from build123d import *

# Parameters (mm, degrees)
SKETCH1_W                                           = 125
SKETCH1_H                                           = 20
BOSS_EXTRUDE1_DEPTH                                 = 32
SKETCH2_R                                           = 6.4897
CUT_EXTRUDE1_DEPTH                                  = 4
SKETCH3_R                                           = 6.5
CUT_EXTRUDE2_DEPTH                                  = 6.5
CUT_EXTRUDE4_REACH                                  = 132.572
SKETCH8_R                                           = 2.1
SKETCH9_R                                           = 2.825
CUT_EXTRUDE5_DEPTH                                  = 1.1
M3X0_5_TAPPED_HOLE1_AT_2_COUNT                      = 2
M3X0_5_TAPPED_HOLE1_AT_2_PITCH                      = 14
LPATTERN1_COUNT                                     = 5
LPATTERN1_PITCH                                     = 25
M2_TAPPED_HOLE1_REACH                               = 132.572
M2_TAPPED_HOLE1_BORE_R                              = 0.8
CBORE_FOR_M6_HEX_SOCKET_HEAD_CAP_SCREW1_D           = 6.2
CBORE_FOR_M6_HEX_SOCKET_HEAD_CAP_SCREW1_CBORE_D     = 10.5
CBORE_FOR_M6_HEX_SOCKET_HEAD_CAP_SCREW1_CBORE_DEPTH = 4


with BuildPart() as part:
    # Sketch1 → Boss-Extrude1 (new body)
    with BuildSketch(Plane(origin=(0, 0, 0), x_dir=(1, 0, 0), z_dir=(0, 1, 0))):
        with Locations((62.5, 10)):
            Rectangle(SKETCH1_W, SKETCH1_H)
    extrude(amount=BOSS_EXTRUDE1_DEPTH)

    # Sketch2 → Cut-Extrude1 (cut)
    with BuildSketch(Plane.XY):
        with Locations((12.5, 16)):
            Circle(SKETCH2_R)
    cut_extrude1 = extrude(amount=-CUT_EXTRUDE1_DEPTH, mode=Mode.SUBTRACT)

    # Sketch3 → Cut-Extrude2 (cut)
    with BuildSketch(Plane.XY.offset(-4)):
        with Locations((12.5, 16)):
            Circle(SKETCH3_R)
    cut_extrude2 = extrude(amount=-CUT_EXTRUDE2_DEPTH, mode=Mode.SUBTRACT)

    # Sketch6 → M12x0.5 Tapped Hole1 (revolve, cut)
    with BuildSketch(Plane(origin=(12.5, 16, -10.5), x_dir=(0, -1, 0), z_dir=(1, 0, 0))):
        Polygon((0, 0), (0, 7.454948559), (5.75, 4), (5.75, 0), align=None)
    m12x0_5_tapped_hole1 = revolve(axis=Axis((12.5, 16, -4.15), (0, 0, -1)), mode=Mode.SUBTRACT)

    # Sketch8 → Cut-Extrude4 (cut, up to next)
    with BuildSketch(Plane.XY, mode=Mode.PRIVATE) as cut_extrude4_sk1:
        with Locations((12.5, 16)):
            Circle(SKETCH8_R)
    cut_extrude4_tool1 = extrude(cut_extrude4_sk1.sketch, amount=-CUT_EXTRUDE4_REACH, mode=Mode.PRIVATE) & part.part
    cut_extrude4 = cut_extrude4_tool1.solids().sort_by_distance((12.5, 16, 0))[0]
    add(cut_extrude4, mode=Mode.SUBTRACT)

    # Sketch9 → Cut-Extrude5 (cut)
    with BuildSketch(Plane(origin=(0, 0, -20), x_dir=(-1, 0, 0), z_dir=(0, 0, -1))):
        with Locations((-12.5, 16)):
            Circle(SKETCH9_R)
    cut_extrude5 = extrude(amount=-CUT_EXTRUDE5_DEPTH, mode=Mode.SUBTRACT)

    # Sketch11 → M3x0.5 Tapped Hole1 (revolve, cut)
    with BuildSketch(Plane(origin=(19.5, 16, -20), x_dir=(0, 1, 0), z_dir=(1, 0, 0))):
        Polygon((0, 0), (0, 5.251075774), (1.25, 4.5), (1.25, 0), align=None)
    m3x0_5_tapped_hole1 = revolve(axis=Axis((19.5, 16, -26.35), (0, 0, 1)), mode=Mode.SUBTRACT)

    # M3x0.5 Tapped Hole1 at 2: M3x0.5 Tapped Hole1 ×2
    with Locations(*[(-i * M3X0_5_TAPPED_HOLE1_AT_2_PITCH, 0, 0) for i in range(1, M3X0_5_TAPPED_HOLE1_AT_2_COUNT)]):
        add(m3x0_5_tapped_hole1, mode=Mode.SUBTRACT)

    # LPattern1: Cut-Extrude1, Cut-Extrude2, M12x0.5 Tapped Hole1, Cut-Extrude4, Cut-Extrude5, M3x0.5 Tapped Hole1 ×5
    with Locations(*[(i * LPATTERN1_PITCH, 0, 0) for i in range(1, LPATTERN1_COUNT)]):
        add(cut_extrude1, mode=Mode.SUBTRACT)
        add(cut_extrude2, mode=Mode.SUBTRACT)
        add(m12x0_5_tapped_hole1, mode=Mode.SUBTRACT)
        add(cut_extrude4, mode=Mode.SUBTRACT)
        add(cut_extrude5, mode=Mode.SUBTRACT)
        add(m3x0_5_tapped_hole1, mode=Mode.SUBTRACT)

    # LPattern1 copy 1 sketch → LPattern1 copy 1 (revolve, cut)
    with BuildSketch(Plane(origin=(30.5, 16, -20), x_dir=(0, 1, 0), z_dir=(1, 0, 0))):
        Polygon((0, 0), (0, 5.251075774), (1.25, 4.5), (1.25, 0), align=None)
    revolve(axis=Axis((30.5, 16, -26.35), (0, 0, 1)), mode=Mode.SUBTRACT)

    # LPattern1 copy 2 sketch → LPattern1 copy 2 (revolve, cut)
    with BuildSketch(Plane(origin=(55.5, 16, -20), x_dir=(0, 1, 0), z_dir=(1, 0, 0))):
        Polygon((0, 0), (0, 5.251075774), (1.25, 4.5), (1.25, 0), align=None)
    revolve(axis=Axis((55.5, 16, -26.35), (0, 0, 1)), mode=Mode.SUBTRACT)

    # LPattern1 copy 3 sketch → LPattern1 copy 3 (revolve, cut)
    with BuildSketch(Plane(origin=(80.5, 16, -20), x_dir=(0, 1, 0), z_dir=(1, 0, 0))):
        Polygon((0, 0), (0, 5.251075774), (1.25, 4.5), (1.25, 0), align=None)
    revolve(axis=Axis((80.5, 16, -26.35), (0, 0, 1)), mode=Mode.SUBTRACT)

    # LPattern1 copy 4 sketch → LPattern1 copy 4 (revolve, cut)
    with BuildSketch(Plane(origin=(105.5, 16, -20), x_dir=(0, 1, 0), z_dir=(1, 0, 0))):
        Polygon((0, 0), (0, 5.251075774), (1.25, 4.5), (1.25, 0), align=None)
    revolve(axis=Axis((105.5, 16, -26.35), (0, 0, 1)), mode=Mode.SUBTRACT)

    # M2 Tapped Hole1 bore → M2 Tapped Hole1 (cut, up to next)
    with BuildSketch(Plane(origin=(0, 32, 0), x_dir=(1, 0, 0), z_dir=(0, 1, 0)), mode=Mode.PRIVATE) as m2_tapped_hole1_sk1:
        with Locations((12.5, 8.5)):
            Circle(M2_TAPPED_HOLE1_BORE_R)
    m2_tapped_hole1_tool1 = extrude(m2_tapped_hole1_sk1.sketch, amount=-M2_TAPPED_HOLE1_REACH, mode=Mode.PRIVATE) & part.part
    # M2 Tapped Hole1 bore → M2 Tapped Hole1 (cut, up to next)
    with BuildSketch(Plane(origin=(0, 32, 0), x_dir=(1, 0, 0), z_dir=(0, 1, 0)), mode=Mode.PRIVATE) as m2_tapped_hole1_sk2:
        with Locations((37.5, 8.5)):
            Circle(M2_TAPPED_HOLE1_BORE_R)
    m2_tapped_hole1_tool2 = extrude(m2_tapped_hole1_sk2.sketch, amount=-M2_TAPPED_HOLE1_REACH, mode=Mode.PRIVATE) & part.part
    # M2 Tapped Hole1 bore → M2 Tapped Hole1 (cut, up to next)
    with BuildSketch(Plane(origin=(0, 32, 0), x_dir=(1, 0, 0), z_dir=(0, 1, 0)), mode=Mode.PRIVATE) as m2_tapped_hole1_sk3:
        with Locations((62.5, 8.5)):
            Circle(M2_TAPPED_HOLE1_BORE_R)
    m2_tapped_hole1_tool3 = extrude(m2_tapped_hole1_sk3.sketch, amount=-M2_TAPPED_HOLE1_REACH, mode=Mode.PRIVATE) & part.part
    # M2 Tapped Hole1 bore → M2 Tapped Hole1 (cut, up to next)
    with BuildSketch(Plane(origin=(0, 32, 0), x_dir=(1, 0, 0), z_dir=(0, 1, 0)), mode=Mode.PRIVATE) as m2_tapped_hole1_sk4:
        with Locations((87.5, 8.5)):
            Circle(M2_TAPPED_HOLE1_BORE_R)
    m2_tapped_hole1_tool4 = extrude(m2_tapped_hole1_sk4.sketch, amount=-M2_TAPPED_HOLE1_REACH, mode=Mode.PRIVATE) & part.part
    # M2 Tapped Hole1 bore → M2 Tapped Hole1 (cut, up to next)
    with BuildSketch(Plane(origin=(0, 32, 0), x_dir=(1, 0, 0), z_dir=(0, 1, 0)), mode=Mode.PRIVATE) as m2_tapped_hole1_sk5:
        with Locations((112.5, 8.5)):
            Circle(M2_TAPPED_HOLE1_BORE_R)
    m2_tapped_hole1_tool5 = extrude(m2_tapped_hole1_sk5.sketch, amount=-M2_TAPPED_HOLE1_REACH, mode=Mode.PRIVATE) & part.part
    add(m2_tapped_hole1_tool1.solids().sort_by_distance((12.5, 32, -8.5))[0], mode=Mode.SUBTRACT)
    add(m2_tapped_hole1_tool2.solids().sort_by_distance((37.5, 32, -8.5))[0], mode=Mode.SUBTRACT)
    add(m2_tapped_hole1_tool3.solids().sort_by_distance((62.5, 32, -8.5))[0], mode=Mode.SUBTRACT)
    add(m2_tapped_hole1_tool4.solids().sort_by_distance((87.5, 32, -8.5))[0], mode=Mode.SUBTRACT)
    add(m2_tapped_hole1_tool5.solids().sort_by_distance((112.5, 32, -8.5))[0], mode=Mode.SUBTRACT)

    # CBORE for M6 Hex Socket Head Cap Screw1 (through all)
    with Locations(Plane(origin=(0, 32, 0), x_dir=(1, 0, 0), z_dir=(0, 1, 0))):
        with Locations((25, 10), (100, 10)):
            CounterBoreHole(CBORE_FOR_M6_HEX_SOCKET_HEAD_CAP_SCREW1_D / 2, CBORE_FOR_M6_HEX_SOCKET_HEAD_CAP_SCREW1_CBORE_D / 2, CBORE_FOR_M6_HEX_SOCKET_HEAD_CAP_SCREW1_CBORE_DEPTH)


solid = part.part
Build history of the part. All positions in model axes, mm. A direction names the side the tool comes from. Round coordinates to 2 decimals unless told otherwise and drop trailing zeros. Write each loop counter-clockwise with the first axis right and the second up, starting at its lowest first coordinate (ties: lowest second). Pieces come first, ordered by that corner, then holes. Notation, with made-up numbers: M 18,11.25 L 29,11.25 A27 cw 29,39.25 Z; hole C 73,9.25 d1. An arc over 180 degrees is marked long. Answer in a Markdown table with one row per item.
1. Saw through at C-C (z = -1.5). List the corners of the cut face in (x, y).
Geometry check:
| item | result |
|---|---|
| outline | M 0,0 L 125,0 L 125,32 L 0,32 Z; hole C 12.5,16 d12.98; hole C 37.5,16 d12.98; hole C 62.5,16 d12.98; hole C 87.5,16 d12.98; hole C 112.5,16 d12.98 |
2. Saw through at A-A (x = 100). List the corners of the cut face in (y, z), and give its area (3 significant figures).
Geometry check:
| item | result |
|---|---|
| outline | M 0,-20 L 32,-20 L 32,-15.25 L 28,-15.25 L 28,-13.1 L 0,-13.1 Z; M 0,-6.9 L 28,-6.9 L 28,-4.75 L 32,-4.75 L 32,0 L 0,0 Z |
| area | 424 mm2 |
3. Mould opens along X. For faces 1 (the face through (109.805, 16.849, -19.458)), 2 (the face through (125, 16, -10)) say: +X half, -X half, draft (parallel to the pull), parting line (faces both ways), or undercut.
Geometry check:
| item | result |
|---|---|
| face 1 | undercut |
| face 2 | +X half |
4. Flat gauge pins, fed straight in: P1, Ø4.5, axis at x = 12.5, y = 16, coming from the -Z side; P2, Ø4, axis at x = 62.5, y = 16, coming from the +Z side; P3, Ø4, axis at x = 88, y = 14, coming from the +Z side; P4, Ø10.5, axis at x = 87.5, y = 16, coming from the +Z side. Where does each tip first touch, or does it go through?
Geometry check:
| item | result |
|---|---|
| P1 | z = -18.9 |
| P2 | through |
| P3 | z = -15.51 |
| P4 | z = -14.8 |
5. Which spindle directions (+Z, -Z, +X, -X, +Y, -Y) get a long thin tool onto all of the face, cutting with end or side? Do faces 3 (the face through (105, 30, -11.6)), 4 (the face through (93.7, 17.95, -7.2)), 5 (the face through (39.58, 17.91, -19.46)). Say none if no direction does.
Geometry check:
| item | result |
|---|---|
| face 3 | +Y |
| face 4 | +Z |
| face 5 | -Z |
6. Saw through at B-B (y = 26.5). List the corners of the cut face in (x, z).
Geometry check:
| item | result |
|---|---|
| outline | M 0,-20 L 125,-20 L 125,0 L 0,0 Z; hole C 12.5,-8.5 d1.6; hole C 25,-10 d6.2; hole C 37.5,-8.5 d1.6; hole C 62.5,-8.5 d1.6; hole C 87.5,-8.5 d1.6; hole C 100,-10 d6.2; hole C 112.5,-8.5 d1.6 |
7. Probe L1, parallel to X at y = 26, z = -11.5; L2, parallel to X at y = 20, z = -14; L3, parallel to Y at x = 112.5, z = -19.4 (3 decimals). List the from-to ranges inside material, lowest first. Write a range as [from, to].
Geometry check:
| item | result |
|---|---|
| L1 | [0, 22.29], [27.71, 97.29], [102.71, 125] |
| L2 | [0, 8.37], [16.63, 33.37], [41.63, 58.37], [66.63, 83.37], [91.63, 108.37], [116.63, 125] |
| L3 | [0, 13.175], [18.825, 32] |
8. Saw through at D-D (y = 8). List the corners of the cut face in (x, z), and give its area (3 significant figures).
Geometry check:
| item | result |
|---|---|
| outline | M 0,-20 L 125,-20 L 125,0 L 0,0 Z; hole C 25,-10 d6.2; hole C 100,-10 d6.2 |
| area | 2,440 mm2 |
